Geometry: final body of the model. Coordinates: model frame, mm. Round coordinates to 2 decimals unless told otherwise and drop trailing zeros. Loops run counter-clockwise (first coordinate to the right, second up) from the corner with the lowest first, then second, coordinate; pieces in that order, holes last. Notation, with made-up numbers: (86, 5) - (98, 5) arc R37 cw to (98, 44) - close; hole circle Ø1 at (67.25, 61.5). An arc over 180 degrees is marked (long way). Return JSON: item names as keys, results as strings. Group by question number.
1. Material intervals for probe 1 along X at (y, z) = (3.9, 0); probe 2 along X at (y, z) = (2.4, 0); probe 3 along Z at (x, y) = (21.5, 1.4), sorted ascending.
2. Section B-B on x = 0. Return loops of the section in (y, z), and give its area (3 significant figures).
3. Section C-C on y = 1.05. Return loops of the section in (x, z), and give its area (3 significant figures).
4. First-contact query: pin 1 Ø25 at (x, z) = (-5.5, -9) entering from -Y. Flat tip, straight axial feed; report the tip coordinate or a pass-through.
5. Section A-A on z = 0. Return loops of the section in (x, y), and give its area (3 significant figures).
from build123d import *

# Parameters (mm, degrees)
SKIZZE1_W                       = 57
SKIZZE1_H                       = 57
SKIZZE1_R                       = 25.25
AUFSATZ_LINEAR_AUSTRAGEN1_DEPTH = 3.4
AUFSATZ_LINEAR_START            = 3.4
SKIZZE1_3_W                     = 57
SKIZZE1_3_H                     = 57
SKIZZE1_3_R                     = 25.25
SKIZZE1_3_R_2                   = 22.5
AUFSATZ_LINEAR_AUSTRAGEN2_DEPTH = 1.2


with BuildPart() as part:
    # Skizze1 → Aufsatz-Linear austragen1 (new body)
    with BuildSketch(Plane(origin=(0, 0, 0), x_dir=(1, 0, 0), z_dir=(0, 1, 0))):
        Rectangle(SKIZZE1_W, SKIZZE1_H)
        with Locations(Location((0, 0, 0), (0, 0, 270))):
            Circle(SKIZZE1_R, mode=Mode.SUBTRACT)
    extrude(amount=AUFSATZ_LINEAR_AUSTRAGEN1_DEPTH)

    # Skizze1<3> → Aufsatz-Linear austragen2 (add)
    # profile 1 of 2: a face of its own
    with BuildSketch(Plane(origin=(0, 0, 0), x_dir=(1, 0, 0), z_dir=(0, 1, 0)).offset(AUFSATZ_LINEAR_START)):
        Rectangle(SKIZZE1_3_W, SKIZZE1_3_H)
        with Locations(Location((0, 0, 0), (0, 0, 270))):
            Circle(SKIZZE1_3_R, mode=Mode.SUBTRACT)
    # profile 2 of 2: a face of its own
    with BuildSketch(Plane(origin=(0, 0, 0), x_dir=(1, 0, 0), z_dir=(0, 1, 0)).offset(AUFSATZ_LINEAR_START)):
        with Locations(Location((0, 0, 0), (0, 0, 270))):
            Circle(SKIZZE1_3_R)
        with Locations(Location((0, 0, 0), (0, 0, 270))):
            Circle(SKIZZE1_3_R_2, mode=Mode.SUBTRACT)
    extrude(amount=AUFSATZ_LINEAR_AUSTRAGEN2_DEPTH)


solid = part.part
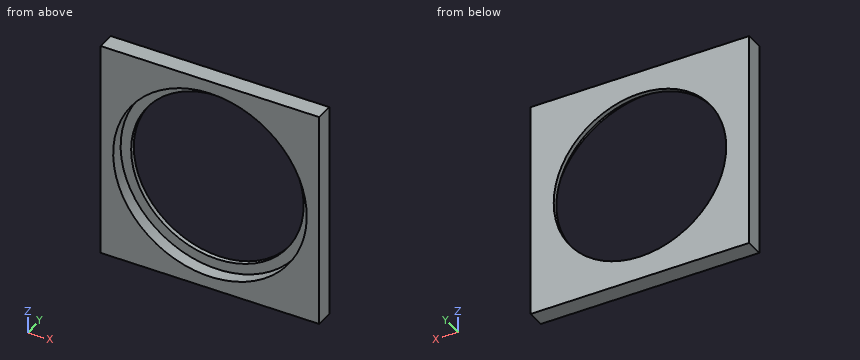
Taken from the geometry:
{
 "1": {"probe 1": "-28.5 to -22.5, 22.5 to 28.5", "probe 2": "-28.5 to -25.25, 25.25 to 28.5", "probe 3": "-28.5 to -13.24, 13.24 to 28.5"},
 "2": {"outline": "(0, -28.5) - (4.6, -28.5) - (4.6, -22.5) - (3.4, -22.5) - (3.4, -25.25) - (0, -25.25) - close; (0, 25.25) - (3.4, 25.25) - (3.4, 22.5) - (4.6, 22.5) - (4.6, 28.5) - (0, 28.5) - close", "area": "36.5 mm2"},
 "3": {"outline": "(-28.5, -28.5) - (28.5, -28.5) - (28.5, 28.5) - (-28.5, 28.5) - close; hole circle Ø50.5 at (0, 0)", "area": "1,250 mm2"},
 "4": {"pin 1": "y = 3.4"},
 "5": {"outline": "(-28.5, 0) - (-25.25, 0) - (-25.25, 3.4) - (-22.5, 3.4) - (-22.5, 4.6) - (-28.5, 4.6) - close; (22.5, 3.4) - (25.25, 3.4) - (25.25, 0) - (28.5, 0) - (28.5, 4.6) - (22.5, 4.6) - close", "area": "36.5 mm2"}
}
